```python
from build123d import *

# Parameters (mm, degrees)
BOSS_EXTRUDE1_DEPTH = 10
CUT_EXTRUDE3_REACH  = 312.322
SKETCH6_W           = 166.922568412
SKETCH6_H           = 253.34709858
BOSS_EXTRUDE2_DEPTH = 10
SKETCH11_R          = 15
BOSS_EXTRUDE4_DEPTH = 9
BOSS_EXTRUDE4_DRAFT = -1
FILLET1_R           = 10
SKETCH15_R          = 11.5
CUT_EXTRUDE6_DEPTH  = 7
SKETCH17_R          = 15
CUT_EXTRUDE7_DEPTH  = 2
CUT_EXTRUDE8_DEPTH  = 1
SKETCH19_R          = 11.05
CUT_EXTRUDE9_DEPTH  = 7
CUT_EXTRUDE10_DEPTH = 10
FILLET2_R           = 2
CUT_EXTRUDE11_DEPTH = 10
FILLET3_R           = 10


with BuildPart() as part:
    # Sketch2 → Boss-Extrude1 (new body)
    with BuildSketch(Plane.XY):
        with BuildLine():
            Line((0, 0), (70, 0))
            ThreePointArc((70, 0), (80.047115298, 146.372811683), (110, 290))
            Line((110, 290), (50, 290))
            ThreePointArc((50, 290), (12.591539765, 147.139389696), (0, 0))
        make_face()
    extrude(amount=BOSS_EXTRUDE1_DEPTH)

    # Sketch6 → Cut-Extrude3 (cut, up to next)
    with BuildSketch(Plane.XY.offset(10), mode=Mode.PRIVATE) as cut_extrude3_sk1:
        with Locations((50.25677389, 83.32645071)):
            Rectangle(SKETCH6_W, SKETCH6_H)
    cut_extrude3_tool1 = extrude(cut_extrude3_sk1.sketch, amount=-CUT_EXTRUDE3_REACH, mode=Mode.PRIVATE) & part.part
    add(cut_extrude3_tool1.solids().sort_by_distance((50.256774, 83.326451, 10))[0], mode=Mode.SUBTRACT)

    # Sketch8 → Boss-Extrude2 (add)
    with BuildSketch(Plane.XY.offset(10)):
        Polygon((25.847632867, 210), (45.521845529, 146.858679142), (90.78507317, 210), align=None)
    extrude(amount=-BOSS_EXTRUDE2_DEPTH)


with BuildPart() as boss_extrude4_tool:
    # Sketch11 → Boss-Extrude4 (with draft: the straight prism first)
    with BuildSketch(Plane.XY.offset(10)):
        with Locations((45.521845529, 146.858679142)):
            Circle(SKETCH11_R)
    extrude(amount=-BOSS_EXTRUDE4_DEPTH)
    # Boss-Extrude4: the draft: its side faces are tilted about the plane it starts from
    boss_extrude4_sides = [boss_extrude4_tool.faces().sort_by_distance(p)[0] for p in [
        (30.521845529, 146.858679142, 5.5),
    ]]
    draft(boss_extrude4_sides, Plane.XY.offset(10), BOSS_EXTRUDE4_DRAFT)


with BuildPart() as part_1:
    add(part.part)

    # Boss-Extrude4: add boss_extrude4_tool
    add(boss_extrude4_tool.part)

    # Fillet1
    fillet1_edges = [part_1.edges().sort_by_distance(p)[0] for p in [
        (25.847632867, 210, 5),
        (90.78507317, 210, 5),
    ]]
    fillet(fillet1_edges, radius=FILLET1_R)

    # Sketch15 → Cut-Extrude6 (cut, symmetric)
    with BuildSketch(Plane(origin=(0, 0, 1), x_dir=(-1, 0, 0), z_dir=(0, 0, -1))):
        with Locations((-45.521845529, 146.858679142)):
            Circle(SKETCH15_R)
    extrude(amount=CUT_EXTRUDE6_DEPTH, both=True, mode=Mode.SUBTRACT)

    # Sketch17 → Cut-Extrude7 (cut)
    with BuildSketch(Plane(origin=(0, 0, 1), x_dir=(-1, 0, 0), z_dir=(0, 0, -1))):
        with Locations((-45.521845529, 146.858679142)):
            Circle(SKETCH17_R)
    extrude(amount=CUT_EXTRUDE7_DEPTH, mode=Mode.SUBTRACT)

    # Sketch18 → Cut-Extrude8 (cut)
    with BuildSketch(Plane.XY.offset(10)):
        with BuildLine():
            Line((83.124410279, 278.596969533), (83.124410279, 292.663120803))
            Line((83.124410279, 292.663120803), (111.699174515, 292.663120803))
            Line((111.699174515, 292.663120803), (111.699174515, 271.967063838))
            Line((111.699174515, 271.967063838), (105.126627558, 271.967063838))
            ThreePointArc((105.126627558, 271.967063838), (91.662229416, 267.107265286), (83.124410279, 278.596969533))
        make_face()
    extrude(amount=-CUT_EXTRUDE8_DEPTH, mode=Mode.SUBTRACT)

    # Sketch19 → Cut-Extrude9 (cut)
    with BuildSketch(Plane.XY.offset(9)):
        with Locations((95.124410279, 278.596969533)):
            Circle(SKETCH19_R)
    extrude(amount=-CUT_EXTRUDE9_DEPTH, mode=Mode.SUBTRACT)

    # Sketch21 → Cut-Extrude10 (cut)
    with BuildSketch(Plane.XY.offset(9)):
        with BuildLine():
            Line((83.124410279, 278.596969533), (83.124410279, 291.961474959))
            Line((83.124410279, 291.961474959), (91.38664408, 291.961474959))
            Line((91.38664408, 291.961474959), (91.38664408, 290))
            ThreePointArc((91.38664408, 290), (85.407075398, 285.63780775), (83.124410279, 278.596969533))
        make_face()
        with BuildLine():
            Line((97.418656909, 290.449512128), (97.418656909, 291.961474959))
            Line((97.418656909, 291.961474959), (113.129922851, 291.961474959))
            Line((113.129922851, 291.961474959), (113.129922851, 278.596969533))
            Line((113.129922851, 278.596969533), (107.196954898, 278.596969533))
            ThreePointArc((107.196954898, 278.596969533), (104.436867753, 286.279707937), (97.418656909, 290.449512128))
        make_face()
    extrude(amount=-CUT_EXTRUDE10_DEPTH, mode=Mode.SUBTRACT)

    # Fillet2
    fillet2_edges = [part_1.edges().sort_by_distance(p)[0] for p in [
        (83.124410279, 278.596969533, 4.5),
    ]]
    fillet(fillet2_edges, radius=FILLET2_R)

    # Sketch22 → Cut-Extrude11 (cut)
    with BuildSketch(Plane.XY.offset(10)):
        Polygon((60, 290), (29.380219364, 191.412034288), (8.711867435, 204.425441059), (44.690109682, 301.643244577), align=None)
    extrude(amount=-CUT_EXTRUDE11_DEPTH, mode=Mode.SUBTRACT)

    # Fillet3
    fillet3_edges = [part_1.edges().sort_by_distance(p)[0] for p in [
        (30.508011562, 195.04324053, 5),
    ]]
    fillet(fillet3_edges, radius=FILLET3_R)


solid = part_1.part
```
Work out the finished part from the listing and answer in its coordinate system (mm). A direction names the side the tool comes from. Round coordinates to 2 decimals unless told otherwise and drop trailing zeros. Write each loop counter-clockwise with the first axis right and the second up, starting at its lowest first coordinate (ties: lowest second). Pieces come first, ordered by that corner, then holes.
1) A cutting plane is placed at A-A on z = 6. Determine the outline of the cut face in (x, y), and give its area (3 significant figures).
2) Consider probe 1 along Y at (x, z) = (89.5, 5); probe 2 along Y at (x, z) = (88, 2.75); probe 3 along X at (y, z) = (149, 9.5). Determine where each line is inside the solid, lowest interval first.
3) Which of the six approach directions +Z, -Z, +X, -X, +Y, -Y give full straight-line access (tool end or side, diameter ignored) to faces 4 (the face through (101.065, 287.914, 5.549)), 5 (the face through (98.52, 245.54, 4.93)), 6 (the face through (88.823, 288.81, 4.563)), 7 (the face through (89, 288, 9)), 8 (the face through (46, 147, 8))?
4) Flat-ended cylindrical pins translate along their axes: P1, Ø4, axis at x = 83.5, z = 4.5, coming from the -Y side; P2, Ø20.5, axis at x = 45.52, y = 146.86, coming from the -Z side; P3, Ø9, axis at x = 44, y = 154, coming from the -Z side; P4, Ø1, axis at x = 62, y = 148.5, coming from the -Z side. Find the tip coordinate at first contact, or state that the pin passes through.
5) A cutting plane is placed at B-B on y = 269.5. Determine the outline of the cut face in (x, z), and give its area (3 significant figures).
6) A cutting plane is placed at C-C on x = 71.5. Determine the outline of the cut face in (y, z).
7) A cutting plane is placed at D-D on y = 233. Determine the outline of the cut face in (x, z).
8) Determine the mould class of faces 1 (the face through (90.56, 210.06, 4.93)), 2 (the face through (42.594, 132.226, 5.563)), 3 (the face through (69, 225, 0)) for opening direction Y: pulls with the +Y half, pulls with the -Y half, needs draft (parallel to the pull), parting line crosses it, or undercut.
Entries:
1. outline: (31.43, 192.07) - (41.08, 161.11) arc R14.93 ccw (long way) to (54.22, 158.99) - (89.53, 208.25) arc R10 ccw to (91.21, 212.1) arc R1071.25 cw to (107.15, 279.67) arc R12.07 ccw to (99.09, 290) - (91.39, 290) arc R12 ccw to (86.55, 287) arc R2 cw to (83.12, 288.39) - (83.12, 290) - (60, 290) - (31.43, 198.01) arc R10 ccw to start; hole circle Ø23 at (45.52, 146.86); hole circle Ø22.1 at (95.12, 278.6)
1. area: 5,900 mm2
2. probe 1: y = 208.21 to 269.09, 288.11 to 289.2
2. probe 2: y = 206.11 to 270.15, 287.04 to 288.25
2. probe 3: x = 30.68 to 60.36
3. face 4: +Z
3. face 5: +Z, -Z, +X, -Y
3. face 6: +Z, -Z, +Y
3. face 7: +Z, +Y
3. face 8: -Z
4. P1: stops at y = 197.05
4. P2: stops at z = 8
4. P3: stops at z = 1
4. P4: passes through
5. outline: (53.63, 0) - (104.45, 0) - (104.45, 10) - (102.95, 10) - (102.95, 9) - (101.4, 9) - (101.4, 2) - (88.85, 2) - (88.85, 9) - (87.3, 9) - (87.3, 10) - (53.63, 10) - close
5. area: 405 mm2
6. outline: (183.1, 0) - (290, 0) - (290, 10) - (183.1, 10) - close
7. outline: (42.3, 0) - (95.65, 0) - (95.65, 10) - (42.3, 10) - close
8. face 1: pulls with the -Y half
8. face 2: undercut
8. face 3: needs draft
